from build123d import *

# Parameters (mm, degrees)
F0_W     = 100
F0_H     = 50
F1_DEPTH = 5
F2_W     = 2
F2_H     = 48
F3_DEPTH = 40
F4_W     = 20
F4_H     = 34
F5_DEPTH = 5
F6_W     = 20
F6_H     = 34
F7_DEPTH = 5
F8_W     = 20
F8_H     = 34
F9_DEPTH = 5


with BuildPart() as f1:
    # F0 (on Top) → F1 (new body)
    with BuildSketch(Plane.XY):
        with Locations((19.01981, 8.886849)):
            Rectangle(F0_W, F0_H)
    extrude(amount=F1_DEPTH)

    # F2 (on face) → F3 (join)
    with BuildSketch(Plane.XY.offset(5)):
        Polygon((-28.98019, 33.886849), (-30.98019, 33.886849), (-30.98019, -16.113151), (-28.98019, -16.113151), (-28.98019, -14.113151), align=None)
        Polygon((67.01981, -14.113151), (-28.98019, -14.113151), (-28.98019, -16.113151), (69.01981, -16.113151), (69.01981, -14.113151), align=None)
        with Locations((68.01981, 9.886849)):
            Rectangle(F2_W, F2_H)
    extrude(amount=F3_DEPTH)

    # F4 (on face) → F5 (cut)
    with BuildSketch(Plane.XZ.offset(16.113151)):
        with Locations((-16.98019, 24)):
            Rectangle(F4_W, F4_H)
        with Locations((7.01981, 24)):
            Rectangle(F4_W, F4_H)
        with Locations((31.01981, 24)):
            Rectangle(F4_W, F4_H)
        with Locations((55.01981, 24)):
            Rectangle(F4_W, F4_H)
    extrude(amount=-F5_DEPTH, mode=Mode.SUBTRACT)

    # F6 (on face) → F7 (cut)
    with BuildSketch(Plane(origin=(-30.98019, 0, 0), x_dir=(0, -1, 0), z_dir=(-1, 0, 0))):
        with Locations((-19.886849, 24)):
            Rectangle(F6_W, F6_H)
        with Locations((2.113151, 24)):
            Rectangle(F6_W, F6_H)
    extrude(amount=-F7_DEPTH, mode=Mode.SUBTRACT)

    # F8 (on face) → F9 (cut)
    with BuildSketch(Plane.YZ.offset(69.01981)):
        with Locations((-2.113151, 24)):
            Rectangle(F8_W, F8_H)
        with Locations((19.886849, 24)):
            Rectangle(F8_W, F8_H)
    extrude(amount=-F9_DEPTH, mode=Mode.SUBTRACT)


solid = f1.part
Model file for the job. Use its own axes, mm. A direction names the side the tool comes from. Coordinates: 2 decimals unless noted, no trailing zeros. Loops run counter-clockwise (first coordinate to the right, second up) from the corner with the lowest first, then second, coordinate; pieces in that order, holes last. Notation, with made-up numbers: (-39.5, -18) -> (-21.5, -18) arc R16 cw to (-21.5, 1) -> close; hole circle Ø2 at (-24, 77). An arc over 180 degrees is marked (long way). Use one line per item in the form item = value. Start each with the question number.
(1) Flat gauge pins, fed straight in: pin 1 (1.5 mm diameter, centred on x = 21.5, z = 21.5, fed in from -Y); pin 2 (12 mm diameter, centred on x = 52, z = 15.5, fed in from +Y); pin 3 (1 mm diameter, centred on x = 48, y = -7.5, fed in from +Z). Where does each tip first touch, or does it go through?
(2) Cut at A-A on x = 5. Give the cut face in (y, z), and give its area (3 significant figures).
(3) Cut at C-C on y = 31.5. Give the cut face in (x, z).
(4) Tool access for faces 3 (the flat face through (-6.98, -15, 24)), 4 (the flat face through (68, 9.887, 24)), 5 (the flat face through (18, 9, 0)), 6 (the flat face through (67.02, 9.6, 24.7)): list every direction of +Z, -Z, +X, -X, +Y, -Y with a clear straight run to the whole face (end or side of a thin tool).
(5) Pull direction X, two halves, no side cores. Call faces 1 (the flat face through (-30, 7.887, 24)), 2 (the flat face through (17.02, -15, 24)): pulls with the +X half, pulls with the -X half, needs draft (parallel to the pull), parting line crosses it, or undercut.
(6) Probe probe 1 along X at (y, z) = (8.5, 13); probe 2 along Z at (x, y) = (43.5, -8); probe 3 along Y at (x, z) = (42, 31.5). List the from-to ranges inside material, lowest first. Write a range as from..to.
(7) Cut at D-D on z = 20. Give the number of separate pieces and of enclosed holes in the cut face, and give its area (3 significant figures).
(8) Cut at B-B on y = -2.5. Give the cut face in (x, z).
Values:
q1.pin_1 = -16.11
q1.pin_2 = through
q1.pin_3 = 5
q2.outline = (-16.11, 0) -> (33.89, 0) -> (33.89, 5) -> (-14.11, 5) -> (-14.11, 7) -> (-16.11, 7) -> close; (-16.11, 41) -> (-14.11, 41) -> (-14.11, 45) -> (-16.11, 45) -> close
q2.area = 262 mm2
q3.outline = (-30.98, 0) -> (69.02, 0) -> (69.02, 45) -> (67.02, 45) -> (67.02, 5) -> (-28.98, 5) -> (-28.98, 45) -> (-30.98, 45) -> close
q4.face_3 = +Y, -Y
q4.face_4 = +X, -X
q4.face_5 = -Z, +X, -X, +Y, -Y
q4.face_6 = +Z, +Y
q5.face_1 = needs draft
q5.face_2 = undercut
q6.probe_1 = -30.98..-28.98, 67.02..69.02
q6.probe_2 = 0..5
q6.probe_3 = -16.11..-14.11
q7.separate_pieces = 9
q7.enclosed_holes = 0
q7.area = 72.0 mm2
q8.outline = (-30.98, 0) -> (69.02, 0) -> (69.02, 7) -> (67.02, 7) -> (67.02, 5) -> (-28.98, 5) -> (-28.98, 7) -> (-30.98, 7) -> close; (-30.98, 41) -> (-28.98, 41) -> (-28.98, 45) -> (-30.98, 45) -> close; (67.02, 41) -> (69.02, 41) -> (69.02, 45) -> (67.02, 45) -> close
